from build123d import *

# Parameters (mm, degrees)
F0_R     = 32
F1_DEPTH = 30


with BuildPart() as f1:
    # F0 (on Front) → F1 (new body)
    with BuildSketch(Plane.XZ):
        with BuildLine():
            Line((-123.021963, 29.088755), (-123.021963, -58.911245))
            Line((-123.021963, -58.911245), (-14.377067, -58.911245))
            Line((-14.377067, -58.911245), (-14.377067, -18.911245))
            Line((-14.377067, -18.911245), (23.978037, -18.911245))
            ThreePointArc((23.978037, -18.911245), (30.128795, -4.062003), (44.978037, 2.088755))
            Line((44.978037, 2.088755), (44.978037, 32.678131))
            Line((44.978037, 32.678131), (116.978037, 32.678131))
            Line((116.978037, 32.678131), (116.978037, 41.088755))
            Line((116.978037, 41.088755), (28.978037, 93.088755))
            Line((28.978037, 93.088755), (-59.021963, 93.088755))
            Line((-59.021963, 93.088755), (-123.021963, 29.088755))
        make_face()
        with Locations((-51.021963, 32.678131)):
            Circle(F0_R, mode=Mode.SUBTRACT)
        with BuildLine():
            Line((-14.377067, -18.911245), (-14.377067, -58.911245))
            Line((-14.377067, -58.911245), (116.978037, -58.911245))
            Line((116.978037, -58.911245), (116.978037, 32.678131))
            Line((116.978037, 32.678131), (44.978037, 32.678131))
            Line((44.978037, 32.678131), (44.978037, 2.088755))
            ThreePointArc((44.978037, 2.088755), (59.827279, -4.062003), (65.978037, -18.911245))
            ThreePointArc((65.978037, -18.911245), (44.978037, -39.911245), (23.978037, -18.911245))
            Line((23.978037, -18.911245), (-14.377067, -18.911245))
        make_face()
    extrude(amount=F1_DEPTH)


solid = f1.part
Source: CAD feature listing. Evaluate the final solid. Frame: model axes, mm. Round coordinates to 2 decimals unless told otherwise and drop trailing zeros. Loops run counter-clockwise (first coordinate to the right, second up) from the corner with the lowest first, then second, coordinate; pieces in that order, holes last.
Q1. Mould query, pull axis X, two halves, no side actions, for faces 1 (the face through (-5, -30, 1)), 2 (the face through (73.594, -14.79, 66.725)), 3 (the face through (-76.42, -14.79, 13.21)), 4 (the face through (-90.57, -14.79, 61.54)). Classes: pulls with the +X half, pulls with the -X half, needs draft (parallel to the pull), parting line crosses it, or undercut.
Q2. First-contact query: P1, Ø1.5, axis at x = -76, y = -7.5, coming from the +Z side; P2, Ø10, axis at x = 64, z = -32.5, coming from the +Y side. Flat tips, straight axial feed; report the tip coordinate or a pass-through.
Q3. Section C-C, the plane y = -6.25. Return loops of the section in (x, z), plus the area to 3 significant figures.
Q4. Ray query, line 1 (Z direction, x = -47.5, y = -1.25); line 2 (X direction, y = -18.25, z = -8); line 3 (Z direction, x = -77, y = -21). Return the intervals inside material, ascending.
Q5. Section D-D, the plane x = -89. Return loops of the section in (y, z), plus the area to 3 significant figures.
Q6. Section A-A, the plane z = 10.5. Return loops of the section in (x, y), plus the area to 3 significant figures.
Q7. Section B-B, the plane x = 60.5. Return loops of the section in (y, z).
Solutions:
1. face 1: needs draft
1. face 2: pulls with the +X half
1. face 3: undercut
1. face 4: pulls with the -X half
2. P1: stops at z = 76.86
2. P2: stops at y = 0
3. outline: (-123.02, -58.91) - (116.98, -58.91) - (116.98, 41.09) - (28.98, 93.09) - (-59.02, 93.09) - (-123.02, 29.09) - close; hole circle Ø64 at (-51.02, 32.68); hole (23.98, -18.91) arc R21 ccw to (65.98, -18.91) arc R21 ccw to (44.98, 2.09) arc R21 ccw to start
3. area: 27,500 mm2
4. line 1: z = -58.91 to 0.87, 64.48 to 93.09
4. line 2: x = -123.02 to 27.04, 62.92 to 116.98
4. line 3: z = -58.91 to 13.99, 51.36 to 75.11
5. outline: (-30, -58.91) - (0, -58.91) - (0, 63.11) - (-30, 63.11) - close
5. area: 3,660 mm2
6. outline: (-123.02, -30) - (-74.09, -30) - (-74.09, 0) - (-123.02, 0) - close; (-27.95, -30) - (116.98, -30) - (116.98, 0) - (-27.95, 0) - close
6. area: 5,820 mm2
7. outline: (-30, -58.91) - (0, -58.91) - (0, -33.06) - (-30, -33.06) - close; (-30, -4.77) - (0, -4.77) - (0, 74.46) - (-30, 74.46) - close
